CAD build for the part. Positions are in the model's coordinates, mm. Face numbers are marked on the shaded views. Give positions to 0.01 mm unless a question says otherwise; leave off trailing zeros. Order: outer loops, then holes, each group sorted by start corner. A loop starts at its lowest first (then second) coordinate and runs counter-clockwise, first axis right, second up.
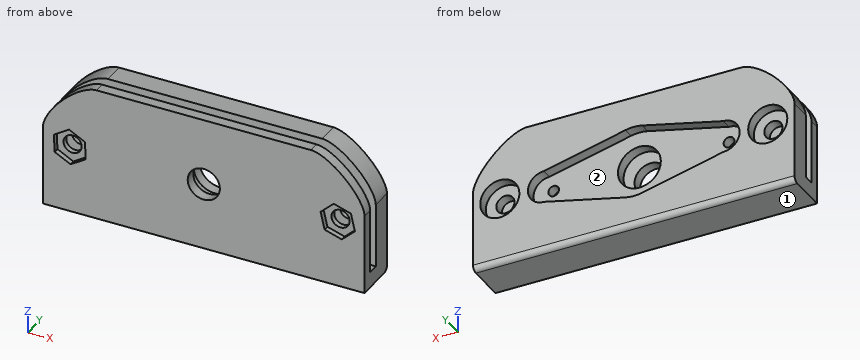
```python
from build123d import *

# Parameters (mm, degrees)
SKETCH1_W           = 60
SKETCH1_H           = 8
BOSS_EXTRUDE1_DEPTH = 25
SKETCH2_W           = 60
SKETCH2_H           = 2
CUT_EXTRUDE1_DEPTH  = 22
CUT_EXTRUDE2_DEPTH  = 2
SKETCH4_R           = 1
SKETCH4_R_2         = 4
CUT_EXTRUDE3_DEPTH  = 2.5
SKETCH5_R           = 1.7
CUT_EXTRUDE4_DEPTH  = 9
FILLET1_R           = 1
FILLET2_SIZE        = 10
SKETCH6_R           = 3
CUT_EXTRUDE5_DEPTH  = 4.5
CUT_EXTRUDE6_DEPTH  = 1
SKETCH8_R           = 3.65
CUT_EXTRUDE7_DEPTH  = 2


with BuildPart() as part:
    # Sketch1 → Boss-Extrude1 (new body)
    with BuildSketch(Plane.XY):
        with Locations((9.92851316, -6.03519833)):
            Rectangle(SKETCH1_W, SKETCH1_H)
    extrude(amount=BOSS_EXTRUDE1_DEPTH)

    # Sketch2 → Cut-Extrude1 (cut)
    with BuildSketch(Plane.XY.offset(25)):
        with Locations((9.92851316, -7.03519833)):
            Rectangle(SKETCH2_W, SKETCH2_H)
    extrude(amount=-CUT_EXTRUDE1_DEPTH, mode=Mode.SUBTRACT)

    # Sketch3 → Cut-Extrude2 (cut)
    with BuildSketch(Plane(origin=(0, -2.03519833, 0), x_dir=(1, 0, 0), z_dir=(0, 1, 0))):
        with BuildLine():
            Line((26.67851316, -9.5), (11.471726674, -5.928775453))
            ThreePointArc((11.471726674, -5.928775453), (9.92851316, -5.75), (8.385299646, -5.928775453))
            Line((8.385299646, -5.928775453), (-6.82148684, -9.5))
            ThreePointArc((-6.82148684, -9.5), (-9.821486841, -12.5), (-6.82148684, -15.5))
            Line((-6.82148684, -15.5), (8.385299646, -19.071224547))
            ThreePointArc((8.385299646, -19.071224547), (9.92851316, -19.25), (11.471726674, -19.071224547))
            Line((11.471726674, -19.071224547), (26.67851316, -15.5))
            ThreePointArc((26.67851316, -15.5), (29.67851316, -12.5), (26.67851316, -9.5))
        make_face()
    extrude(amount=-CUT_EXTRUDE2_DEPTH, mode=Mode.SUBTRACT)

    # Sketch4 → Cut-Extrude3 (cut)
    with BuildSketch(Plane(origin=(0, -4.03519833, 0), x_dir=(1, 0, 0), z_dir=(0, 1, 0))):
        with Locations(Location((-6.796927173, -12.5, 0), (0, 0, 270))):
            Circle(SKETCH4_R)
        with Locations(Location((9.92851316, -12.5, 0), (0, 0, 270))):
            Circle(SKETCH4_R_2)
        with Locations(Location((25.92851316, -12.5, 0), (0, 0, 270))):
            Circle(SKETCH4_R)
    extrude(amount=-CUT_EXTRUDE3_DEPTH, mode=Mode.SUBTRACT)

    # Sketch5 → Cut-Extrude4 (cut)
    with BuildSketch(Plane(origin=(0, -2.03519833, 0), x_dir=(1, 0, 0), z_dir=(0, 1, 0))):
        with Locations(Location((34.92851316, -12.5, 0), (0, 0, 270))):
            Circle(SKETCH5_R)
        with Locations(Location((-15.07148684, -12.5, 0), (0, 0, 270))):
            Circle(SKETCH5_R)
    extrude(amount=-CUT_EXTRUDE4_DEPTH, mode=Mode.SUBTRACT)

    # Fillet1
    fillet1_edges = [part.edges().sort_by_distance(p)[0] for p in [
        (9.92851316, -2.03519833, 0),
    ]]
    fillet(fillet1_edges, radius=FILLET1_R)

    # Fillet2
    # a fillet whose section is not a circle: 10 mm, written as the material it takes off along each edge
    with BuildSketch(Plane(origin=(-20.07148684, -31.03519833, 25), x_dir=(0, 0, -1), z_dir=(0, 1, 0))) as fillet2_piece_1:
        with BuildLine():
            Bezier((FILLET2_SIZE, 0), (0, 0), (0, -FILLET2_SIZE), weights=[1, 0.353553391, 1])
            Line((0, -FILLET2_SIZE), (0, 0))
            Line((0, 0), (FILLET2_SIZE, 0))
        make_face()
    extrude(amount=54, mode=Mode.SUBTRACT)
    with BuildSketch(Plane(origin=(-20.07148684, -35.03519833, 25), x_dir=(0, 0, -1), z_dir=(0, 1, 0)), Plane(origin=(39.92851316, 16.96480167, 25), x_dir=(0, 0, -1), z_dir=(0, -1, 0))) as fillet2_piece_2:
        with BuildLine():
            Bezier((FILLET2_SIZE, 0), (0, 0), (0, -FILLET2_SIZE), weights=[1, 0.353553391, 1])
            Line((0, -FILLET2_SIZE), (0, 0))
            Line((0, 0), (FILLET2_SIZE, 0))
        make_face()
    extrude(amount=52, mode=Mode.SUBTRACT)
    with BuildSketch(Plane(origin=(39.92851316, 22.96480167, 25), x_dir=(-1, 0, 0), z_dir=(0, -1, 0))) as fillet2_piece_3:
        with BuildLine():
            Bezier((FILLET2_SIZE, 0), (0, 0), (0, FILLET2_SIZE), weights=[1, 0.353553391, 1])
            Line((0, FILLET2_SIZE), (0, 0))
            Line((0, 0), (FILLET2_SIZE, 0))
        make_face()
    extrude(amount=54, mode=Mode.SUBTRACT)

    # Sketch6 → Cut-Extrude5 (cut)
    with BuildSketch(Plane(origin=(0, -8.03519833, 0), x_dir=(1, 0, 0), z_dir=(0, 1, 0))):
        with Locations(Location((9.92851316, -12.5, 0), (0, 0, 270))):
            Circle(SKETCH6_R)
    extrude(amount=-CUT_EXTRUDE5_DEPTH, mode=Mode.SUBTRACT)

    # Sketch7 → Cut-Extrude6 (cut)
    with BuildSketch(Plane(origin=(0, -10.03519833, 0), x_dir=(-1, 0, 0), z_dir=(0, -1, 0))):
        Polygon((-35.683884991, -9.237677709), (-38.131453055, -11.52301005), (-37.376081224, -14.785332341), (-34.173141329, -15.762322291), (-31.725573265, -13.47698995), (-32.480945096, -10.214667659), align=None)
        Polygon((12.105656047, -10.945271393), (12.242136974, -14.291120506), (15.207967766, -15.845849113), (18.037317633, -14.054728607), (17.900836706, -10.708879494), (14.935005914, -9.154150887), align=None)
    extrude(amount=-CUT_EXTRUDE6_DEPTH, mode=Mode.SUBTRACT)

    # Sketch8 → Cut-Extrude7 (cut)
    with BuildSketch(Plane(origin=(0, -2.03519833, 0), x_dir=(1, 0, 0), z_dir=(0, 1, 0))):
        with Locations(Location((-15.07148684, -12.5, 0), (0, 0, 270))):
            Circle(SKETCH8_R)
        with Locations(Location((34.92851316, -12.5, 0), (0, 0, 270))):
            Circle(SKETCH8_R)
    extrude(amount=-CUT_EXTRUDE7_DEPTH, mode=Mode.SUBTRACT)


solid = part.part
```
Item 1: Drop flat-ended pins along their axis: pin 1 Ø4 at (x, z) = (0.5, 10.5) entering from +Y; pin 2 Ø4 at (x, z) = (34.93, 12.5) entering from -Y; pin 3 Ø3 at (x, z) = (-15.07, 12.5) entering from +Y; pin 4 Ø4 at (x, y) = (-13, -6) entering from +Z. Give the stop position or say it passes through.
Item 2: Slice it at C-C (y = -7). Give the cut face in (x, z).
Item 3: Slice it at D-D (z = 12.5). State how many separate pieces and enclosed holes the cut face has, and give its area (3 significant figures).
Item 4: Slice it at A-A (z = 7.5). Give the cut face in (x, y).
Item 5: Wall check: L1, parallel to X at y = -2.5, z = 12.25; L2, parallel to X at y = -5.45, z = 12.5; L3, parallel to X at y = -8.6, z = 12.5. Give the ranges that are in metal, low to high.
Item 6: Two-plate mould, pull along X, no slides. Class the marked faces 1 and 2: released by +X, released by -X, zero draft, split by the parting line, or undercut.
Item 7: Slice it at B-B (x = 16). Give the cut face in (y, z), and give its area (3 significant figures).
A:
1. pin 1: stops at y = -4.04
1. pin 2: stops at y = -9.04
1. pin 3: passes through
1. pin 4: stops at z = 24.86
2. outline: (-20.07, 0) - (39.93, 0) - (39.93, 3) - (-20.07, 3) - close
3. separate pieces: 10
3. enclosed holes: 0
3. area: 184 mm2
4. outline: (-20.07, -10.04) - (39.93, -10.04) - (39.93, -8.04) - (-20.07, -8.04) - close; (-20.07, -6.04) - (39.93, -6.04) - (39.93, -2.04) - (18.16, -2.04) - (18.16, -4.04) - (1.69, -4.04) - (1.69, -2.04) - (-20.07, -2.04) - close
5. L1: x = -20.07 to -18.71, -11.43 to -9.81, 29.67 to 31.29, 38.57 to 39.93
5. L2: x = -20.07 to -16.77, -13.37 to -7.8, -5.8 to 5.93, 13.93 to 24.93, 26.93 to 33.23, 36.63 to 39.93
5. L3: x = -20.07 to -16.77, -13.37 to 6.93, 12.93 to 33.23, 36.63 to 39.93
6. face 1: zero draft
6. face 2: undercut
7. outline: (-10.04, 0) - (-3.04, 0) arc R1 ccw to (-2.04, 1) - (-2.04, 6.99) - (-4.04, 6.99) - (-4.04, 18.01) - (-2.04, 18.01) - (-2.04, 25) - (-6.04, 25) - (-6.04, 3) - (-8.04, 3) - (-8.04, 25) - (-10.04, 25) - close
7. area: 134 mm2
